```python
from build123d import *

# Parameters (mm, degrees)
SKETCH8_W              = 609.6
SKETCH8_H              = 171.45
BASE_FLANGE3_DEPTH     = 3.175
SKETCHED_START         = -304.8
SKETCHED_BEND3_DEPTH   = 609.6
SKETCHED_BEND3_2_DEPTH = 609.6
SKETCH19_W             = 609.6
SKETCH19_H             = 6.35
CUT_EXTRUDE1_DEPTH     = 327.160318745


# Read off the part's stored shape, not the designer's step: Sketched Bend3
# Sheet-metal steps are written as plain solids
with BuildPart() as part:
    # Sketch8 → Base-Flange3 (new body)
    with BuildSketch(Plane.XY):
        Rectangle(SKETCH8_W, SKETCH8_H)
    extrude(amount=-BASE_FLANGE3_DEPTH)

    # Sketched Bend3 outline → Sketched Bend3 (cut)
    with BuildSketch(Plane.YZ.offset(SKETCHED_START)):
        with BuildLine():
            ThreePointArc((-7.699656128, -3.175), (-10.191576071, -2.278520157), (-11.541274928, 0))
            Line((-11.541274928, 0), (-85.725, 0))
            Line((-85.725, 0), (-85.725, -3.175))
            Line((-85.725, -3.175), (-7.699656128, -3.175))
        make_face()
    extrude(amount=SKETCHED_BEND3_DEPTH, mode=Mode.SUBTRACT)

    # Sketched Bend3 2 outline → Sketched Bend3 2 (add)
    with BuildSketch(Plane.YZ.offset(SKETCHED_START)):
        with BuildLine():
            Line((-8.436256128, 75.111256128), (-11.611256128, 75.111256128))
            Line((-11.611256128, 75.111256128), (-11.611256128, 0.7366))
            ThreePointArc((-11.611256128, 0.7366), (-11.593721527, 0.366641581), (-11.541274928, 0))
            Line((-11.541274928, 0), (-7.699656128, 0))
            ThreePointArc((-7.699656128, 0), (-8.220510983, 0.215745145), (-8.436256128, 0.7366))
            Line((-8.436256128, 0.7366), (-8.436256128, 75.111256128))
        make_face()
    extrude(amount=SKETCHED_BEND3_2_DEPTH)

    # Sketch19 → Cut-Extrude1 (cut, through all)
    with BuildSketch(Plane(origin=(0, 0, -3.175), x_dir=(-1, 0, 0), z_dir=(0, 0, -1))):
        with Locations((0, 82.55)):
            Rectangle(SKETCH19_W, SKETCH19_H)
    extrude(amount=-CUT_EXTRUDE1_DEPTH, mode=Mode.SUBTRACT)


solid = part.part
```
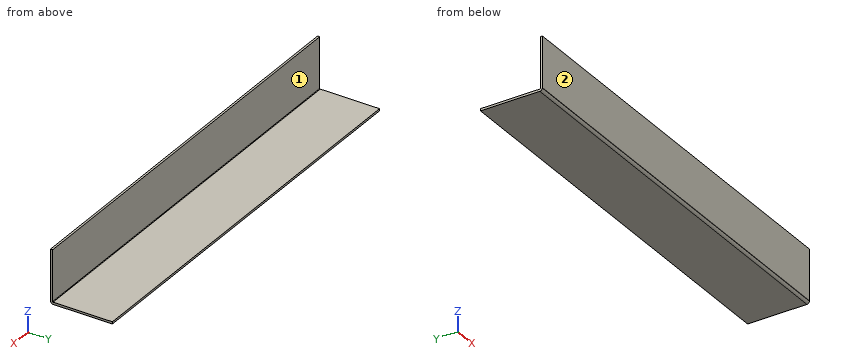
Work out the finished part from the listing and answer in its coordinate system (mm). Face numbers are marked on the shaded views. A direction names the side the tool comes from. Coordinates: 2 decimals unless noted, no trailing zeros. Order: outer loops, then holes, each group sorted by start corner. A loop starts at its lowest first (then second) coordinate and runs counter-clockwise, first axis right, second up. Notation, with made-up numbers: (66.25, 44) - (84.25, 44) arc R23 cw to (84.25, 61) - close; hole circle Ø4 at (5, 6). An arc over 180 degrees is marked (long way). Answer as a JSON object with one key per item and string values.
1. Find section C-C on z = 57. Determine the outline of the cut face in (x, y), plus the area to 3 significant figures.
Output values:
{"outline": "(-304.8, -11.61) - (304.8, -11.61) - (304.8, -8.44) - (-304.8, -8.44) - close", "area": "1,940 mm²"}
2. Consider line 1 (Y direction, x = -65, z = 25); line 2 (Z direction, x = 246.5, y = 61) (3 decimals). Determine where each line is inside the solid, lowest interval first.
Output values:
{"line 1": "y = -11.61 to -8.44", "line 2": "z = -3.175 to 0"}
3. Each of these flat-tipped pins is pushed along its axis until it touches: P1, Ø5, axis at x = 54.5, z = 5, coming from the +Y side; P2, Ø2, axis at x = 137.5, y = 2.5, coming from the +Z side. Where does it stop, or does it pass through?
Output values:
{"P1": "stops at y = -8.44", "P2": "stops at z = 0"}
4. Find section A-A on x = 246.5. Determine the outline of the cut face in (y, z) (3 decimals).
Output values:
{"outline": "(-11.611, 0.737) arc R3.912 ccw to (-7.7, -3.175) - (79.375, -3.175) - (79.375, 0) - (-7.7, 0) arc R0.737 cw to (-8.436, 0.737) - (-8.436, 75.111) - (-11.611, 75.111) - close"}
5. A tool of negligible diameter and unlimited length cuts with its end or side. For the marked faces 1 and 2, from which of +Z, -Z, +X, -X, +Y, -Y can it reach the whole face along a straight path? Write none if from no direction.
Output values:
{"face 1": "+Z, +X, -X, +Y", "face 2": "+Z, -Z, +X, -X, -Y"}
6. Find section B-B on y = 6.5. Determine the outline of the cut face in (x, z) (3 decimals).
Output values:
{"outline": "(-304.8, -3.175) - (304.8, -3.175) - (304.8, 0) - (-304.8, 0) - close"}
